from build123d import *

# Parameters (mm, degrees)
CHANFREIN1_SIZE = 0.5
CONG_1_R        = 0.5


with BuildPart() as part:
    # Esquisse1 → Révolution1 (revolve)
    with BuildSketch(Plane.XY, mode=Mode.PRIVATE) as r_volution1_sk:
        Polygon((0, 56), (5, 56), (5, 50), (3, 50), (3, 25), (2.95, 24.5), (2.95, 0), (0, 0), align=None)
    revolve(r_volution1_sk.sketch.rotate(Axis((0, 0, 0), (0, 1, 0)), 90), axis=Axis((0, 0, 0), (0, 1, 0)))

    # Chanfrein1
    chanfrein1_edges = [part.edges().sort_by_distance(p)[0] for p in [
        (0, 0, 2.95),
    ]]
    chamfer(chanfrein1_edges, length=CHANFREIN1_SIZE)

    # Congé1
    cong_1_edges = [part.edges().sort_by_distance(p)[0] for p in [
        (0, 56, 5),
    ]]
    fillet(cong_1_edges, radius=CONG_1_R)


solid = part.part
Read the model definition and answer for the solid it produces. Units are mm, in the model's axes. A direction names the side the tool comes from. Round coordinates to 2 decimals unless told otherwise and drop trailing zeros. Loops run counter-clockwise (first coordinate to the right, second up) from the corner with the lowest first, then second, coordinate; pieces in that order, holes last.
Q1. Section A-A on z = 0 is taken. Write down the section's boundary in (x, y).
Q2. Section C-C on y = 41 is taken. Write down the section's boundary in (x, z).
Q3. Consider probe 1 along Y at (x, z) = (-3.5, 1); probe 2 along Y at (x, z) = (-3.25, 3.75); probe 3 along Z at (x, y) = (-1.75, 49). Determine where each line is inside the solid, lowest interval first.
Q4. Which of the six approach directions +Z, -Z, +X, -X, +Y, -Y give full straight-line access (tool end or side, diameter ignored) to faces 1 (the face through (0, 0, 0)), 2 (the face through (-0.13, 12.332, 2.947))?
Q5. Each of these flat-tipped pins is pushed along its axis until it touches: pin 1 (6 mm diameter, centred on y = 38.5, z = 1, fed in from +X); pin 2 (2 mm diameter, centred on y = 42, z = -3.5, fed in from -X); pin 3 (5 mm diameter, centred on y = 47, z = -1.5, fed in from -X); pin 4 (4 mm diameter, centred on x = -1.5, z = -3.5, fed in from -Y). Where does it stop, or does it pass through?
Q6. Section B-B on x = 0 is taken. Write down the section's boundary in (y, z), and give its area (3 significant figures).
Output:
1. outline: (-5, 50) - (-3, 50) - (-3, 25) - (-2.95, 24.5) - (-2.95, 0.5) - (-2.45, 0) - (2.45, 0) - (2.95, 0.5) - (2.95, 24.5) - (3, 25) - (3, 50) - (5, 50) - (5, 55.5) arc R0.5 ccw to (4.5, 56) - (-4.5, 56) arc R0.5 ccw to (-5, 55.5) - close
2. outline: circle Ø6 at (0, 0)
3. probe 1: y = 50 to 56
3. probe 2: y = 50 to 55.69
3. probe 3: z = -2.44 to 2.44
4. face 1: +Z, -Z, +X, -X, -Y
4. face 2: -Y
5. pin 1: stops at x = 3
5. pin 2: stops at x = -1.66
5. pin 3: stops at x = -3
5. pin 4: stops at y = 0
6. outline: (0, -2.45) - (0.5, -2.95) - (24.5, -2.95) - (25, -3) - (50, -3) - (50, -5) - (55.5, -5) arc R0.5 ccw to (56, -4.5) - (56, 4.5) arc R0.5 ccw to (55.5, 5) - (50, 5) - (50, 3) - (25, 3) - (24.5, 2.95) - (0.5, 2.95) - (0, 2.45) - close
6. area: 357 mm2
